The listing builds one solid part. Answer for the finished solid, in the listing's coordinates (mm). Coordinates: 2 decimals unless noted, no trailing zeros. Order: outer loops, then holes, each group sorted by start corner. A loop starts at its lowest first (then second) coordinate and runs counter-clockwise, first axis right, second up.
Autodesk Inventor part; units mm, degrees
ref_plane "Work Plane2" through (63.3, 0, 0) normal (1, 0, 0) x (0, 0, -1)
ref_plane "YZ Plane" through (0, 0, 0) normal (1, 0, 0) x (0, 1, 0)
ref_plane "XZ Plane" through (0, 0, 0) normal (0, 1, 0) x (-1, 0, 0)
sketch "Sketch1" plane through (0, 0, 0) normal (0, 0, 1) x (1, 0, 0)
  line L0 (0, 0) -> (126.6, 0)
  line L1 (1.7, 0) -> (1.7, -3.3)
  line L2 (1.7, -3.3) -> (20.7, -3.3)
  line L3 (20.7, -3.3) -> (20.7, 0)
  line L4 (53.35, 0) -> (53.35, -3.3)
  line L5 (53.35, -3.3) -> (73.25, -3.3)
  line L6 (73.25, -3.3) -> (73.25, 0)
  line L7 (105.9, 0) -> (105.9, -3.3)
  line L8 (105.9, -3.3) -> (124.9, -3.3)
  line L9 (124.9, -3.3) -> (124.9, 0)
  line L10 (11.2, -3.3) -> (11.2, 0) construction
  line L11 (63.3, -3.3) -> (63.3, 0) construction
  line L12 (115.4, -3.3) -> (115.4, 0) construction
  line L13 (63.3, 0) -> (63.3, 12.1181) construction
  line L14 (0, 0) -> (0, 58.65)
  line L15 (0, 58.65) -> (126.6, 58.65) construction
  line L16 (126.6, 0) -> (126.6, 58.65)
  line L17 (0, 117.3) -> (126.6, 117.3)
  line L18 (1.7, 117.3) -> (1.7, 120.6)
  line L19 (1.7, 120.6) -> (20.7, 120.6)
  line L20 (20.7, 120.6) -> (20.7, 117.3)
  line L21 (53.35, 117.3) -> (53.35, 120.6)
  line L22 (53.35, 120.6) -> (73.25, 120.6)
  line L23 (73.25, 120.6) -> (73.25, 117.3)
  line L24 (105.9, 117.3) -> (105.9, 120.6)
  line L25 (105.9, 120.6) -> (124.9, 120.6)
  line L26 (124.9, 120.6) -> (124.9, 117.3)
  line L27 (11.2, 120.6) -> (11.2, 117.3) construction
  line L28 (63.3, 120.6) -> (63.3, 117.3) construction
  line L29 (115.4, 120.6) -> (115.4, 117.3) construction
  line L30 (63.3, 117.3) -> (63.3, 105.1819) construction
  line L31 (0, 117.3) -> (0, 58.65)
  line L32 (126.6, 117.3) -> (126.6, 58.65)
  dimension "d12" = 126.6
  dimension "d13" = 3.3
  dimension "d14" = 19
  dimension "d15" = 3.3
  dimension "d16" = 19.9
  dimension "d17" = 3.3
  dimension "d18" = 19
  dimension "d19" = 52.1
  dimension "d20" = 52.1
  dimension "d21" = 58.65
extrude "Extrusion1" add sketch "Sketch1" along normal blind 0.5
ref_plane "Work Plane1" through (0, 0, 0.25) normal (0, 0, 1) x (1, 0, 0)
ref_plane "Work Plane2" through (63.3, 0, 0) normal (1, 0, 0) x (0, 0, -1)
equation "\"d12\" = lrltotal"
equation "\"d13\" = lrdepth"
equation "\"d14\" = lrlr"
equation "\"d15\" = lrdepth"
equation "\"d16\" = lrmid"
equation "\"d17\" = lrdepth"
equation "\"d18\" = lrlr"
equation "\"d20\" = d19"
equation "\"d21\" = 0.5 * heaterH"
equation "\"d22\" = thick"
equation "\"thick\" = 0.5"
equation "\"lrlr\" = 19"
equation "\"lrmid\" = 19.9"
equation "\"lrdepth\" = 3.3"
equation "\"mlr\" = 16.6"
equation "\"mmid\" = 24.7"
equation "\"mdepth\" = 4.5"
equation "\"lrltotal\" = 126.6"
equation "\"mltotal\" = 126.6"
equation "\"lrbetween\" = 52.1"
equation "\"mbetween\" = 49.5"
equation "\"toler\" = 1"
equation "\"stuckw\" = 6"
equation "\"tight\" = 0.08"
equation "\"sidewallL\" = 132.6"
equation "\"heaterH\" = 117.3"
equation "\"stickL\" = 3.5"
equation "\"wireH\" = 25"
properties part number "lr_heater"
1) A cutting plane is placed at A-A, the plane z = 0.4. Write down the section's boundary in (x, y), plus the area to 3 significant figures.
2) A straight line is drawn through the part: probe 1 along Y at (x, z) = (98, 0.15). Find the intervals that lie inside material, in ascending order.
3) This flat-tipped pin is pushed along its axis until it touches: P1, Ø6, axis at x = 50, y = 57, coming from the -Z side. Where does it stop, or does it pass through?
4) A cutting plane is placed at B-B, the plane x = 48. Write down the section's boundary in (y, z).
Working result:
1. outline: (0, 0) - (1.7, 0) - (1.7, -3.3) - (20.7, -3.3) - (20.7, 0) - (53.35, 0) - (53.35, -3.3) - (73.25, -3.3) - (73.25, 0) - (105.9, 0) - (105.9, -3.3) - (124.9, -3.3) - (124.9, 0) - (126.6, 0) - (126.6, 117.3) - (124.9, 117.3) - (124.9, 120.6) - (105.9, 120.6) - (105.9, 117.3) - (73.25, 117.3) - (73.25, 120.6) - (53.35, 120.6) - (53.35, 117.3) - (20.7, 117.3) - (20.7, 120.6) - (1.7, 120.6) - (1.7, 117.3) - (0, 117.3) - close
1. area: 15,200 mm2
2. probe 1: y = 0 to 117.3
3. P1: stops at z = 0
4. outline: (0, 0) - (117.3, 0) - (117.3, 0.5) - (0, 0.5) - close
